Here's how the part is built. I have some questions about the finished solid (model axes, mm). A direction names the side the tool comes from. Coordinates: 2 decimals unless noted, no trailing zeros. Write each loop counter-clockwise with the first axis right and the second up, starting at its lowest first coordinate (ties: lowest second). Pieces come first, ordered by that corner, then holes. Notation, with made-up numbers: (-6, 16.25) -> (5, 16.25) arc R17 cw to (5, 28.25) -> close; hole circle Ø8 at (44.5, 6). An arc over 180 degrees is marked (long way). Put each result on its own line as item: value. Start each with the question number.
Item 1: I want a section at D-D, the plane x = 9. List the corners of the cut face in (y, z) for me, then the cut area to 3 significant figures.
Item 2: If we mould it in two halves opening along Y, with no side actions, what happens to faces 5 (the face through (0, 108, -20)), 6 (the face through (0, 99, -23)), 7 (the face through (0, 15, -8))? For each: released by +Y, released by -Y, zero draft, split by the parting line, or undercut.
Item 3: On a 3-axis mill with a long thin cutter (end or side, diameter ignored), from which of +Z, -Z, +X, -X, +Y, -Y can I reach the whole of each face in a straight line? I mean faces 1 (the face through (20, 35, -16)), 2 (the face through (-17.5, 56, -8)), 3 (the face through (25.65, 102.17, -5.07)), 4 (the face through (-23.34, 53.24, -4.31)). Say none if no direction works.
Item 4: I want a section at B-B, the plane x = 19.5. List the corners of the cut face in (y, z) for me.
Item 5: I want a section at A-A, the plane y = 63.5. List the corners of the cut face in (x, z) for me, then the cut area to 3 significant figures.
Item 6: I need wall thicknesses on line 1 (X direction, y = 100, z = -5); line 2 (X direction, y = 52, z = -4.5); line 3 (X direction, y = 74, z = -10). Which ranges of each line are inside material? Lowest first, please. Write a range as [from, to].
Item 7: I want a section at C-C, the plane y = 10. List the corners of the cut face in (x, z) for me.
Item 8: For pin 1 (4 mm diameter, centred on x = 3.5, z = -36, fed in from -Y); pin 2 (6.5 mm diameter, centred on x = -19.5, y = 10, fed in from -Z), each with a flat end and sliding along its axis, tell me the tip position at first contact or that it passes through.
from build123d import *

# Parameters (mm, degrees)
EXTRUDE_2_DEPTH        = 29.5
HOLE_WIZARD_M4_2_D     = 3.3
HOLE_WIZARD_M4_2_DEPTH = 11.5
HOLE_WIZARD_M4_2_TIP   = 0.991420021
CUT_EXTRUDE_1_DEPTH    = 119.887551914
HOLE_WIZARD_M5_1_D     = 4.2
HOLE_WIZARD_M3_1_D     = 2.5
HOLE_WIZARD_M3_1_DEPTH = 8.5
HOLE_WIZARD_M3_1_TIP   = 0.751075774
HOLE_WIZARD_M4_3_D     = 3.3
HOLE_WIZARD_M4_3_DEPTH = 11.5
HOLE_WIZARD_M4_3_TIP   = 0.991420021


with BuildPart() as part:
    # 草图5 → 凸台-拉伸2 (new, symmetric)
    with BuildSketch(Plane(origin=(0, 0, 0), x_dir=(0, 0, -1), z_dir=(1, 0, 0))):
        Polygon((26, 102), (40, 102), (40, 108), (0, 108), (0, 0), (16, 0), (16, 92), align=None)
    extrude(amount=EXTRUDE_2_DEPTH, both=True)

    # M4 螺纹孔2
    with Locations(Plane(origin=(0, 108, 0), x_dir=(1, 0, 0), z_dir=(0, 1, 0))):
        with Locations((24, 5), (-24, 5)):
            Hole(HOLE_WIZARD_M4_2_D / 2, depth=HOLE_WIZARD_M4_2_DEPTH)
            with Locations((0, 0, -(HOLE_WIZARD_M4_2_DEPTH + HOLE_WIZARD_M4_2_TIP / 2))):  # 118° drill point
                Cone(0, HOLE_WIZARD_M4_2_D / 2, HOLE_WIZARD_M4_2_TIP, mode=Mode.SUBTRACT)

    # 草图8 → 切除-拉伸1 (cut, through all)
    with BuildSketch(Plane.XY):
        with BuildLine():
            Line((17.5, 80.5), (17.5, 32.5))
            ThreePointArc((17.5, 32.5), (0, 15), (-17.5, 32.5))
            Line((-17.5, 32.5), (-17.5, 80.5))
            ThreePointArc((-17.5, 80.5), (0, 98), (17.5, 80.5))
        make_face()
    extrude(amount=-CUT_EXTRUDE_1_DEPTH, mode=Mode.SUBTRACT)

    # M5 螺纹孔1 (through all)
    with Locations(Plane.XY):
        with Locations((-19.5, 10), (19.5, 10)):
            Hole(HOLE_WIZARD_M5_1_D / 2)

    # M3 螺纹孔1
    with Locations(Plane.XY):
        with Locations((23.5, 42), (-23.5, 52), (-23.5, 42), (23.5, 52)):
            Hole(HOLE_WIZARD_M3_1_D / 2, depth=HOLE_WIZARD_M3_1_DEPTH)
            with Locations((0, 0, -(HOLE_WIZARD_M3_1_DEPTH + HOLE_WIZARD_M3_1_TIP / 2))):  # 118° drill point
                Cone(0, HOLE_WIZARD_M3_1_D / 2, HOLE_WIZARD_M3_1_TIP, mode=Mode.SUBTRACT)

    # M4 螺纹孔3
    with Locations(Plane(origin=(0, 0, 0), x_dir=(-1, 0, 0), z_dir=(0, -1, 0))):
        with Locations((0, 8)):
            Hole(HOLE_WIZARD_M4_3_D / 2, depth=HOLE_WIZARD_M4_3_DEPTH)
            with Locations((0, 0, -(HOLE_WIZARD_M4_3_DEPTH + HOLE_WIZARD_M4_3_TIP / 2))):  # 118° drill point
                Cone(0, HOLE_WIZARD_M4_3_D / 2, HOLE_WIZARD_M4_3_TIP, mode=Mode.SUBTRACT)


solid = part.part
Calculated:
1. outline: (0, -16) -> (17.49, -16) -> (17.49, 0) -> (0, 0) -> close; (95.51, -19.51) -> (102, -26) -> (102, -40) -> (108, -40) -> (108, 0) -> (95.51, 0) -> close
1. area: 668 mm2
2. face 5: released by +Y
2. face 6: released by -Y
2. face 7: undercut
3. face 1: -Z, +X, -X, -Y
3. face 2: +Z, -Z
3. face 3: +Y
3. face 4: +Z
4. outline: (0, -16) -> (7.9, -16) -> (7.9, 0) -> (0, 0) -> close; (12.1, -16) -> (92, -16) -> (102, -26) -> (102, -40) -> (108, -40) -> (108, 0) -> (12.1, 0) -> close
5. outline: (-29.5, -16) -> (-17.5, -16) -> (-17.5, 0) -> (-29.5, 0) -> close; (17.5, -16) -> (29.5, -16) -> (29.5, 0) -> (17.5, 0) -> close
5. area: 384 mm2
6. line 1: x = [-29.5, -25.65], [-22.35, 22.35], [25.65, 29.5]
6. line 2: x = [-29.5, -24.75], [-22.25, -17.5], [17.5, 22.25], [24.75, 29.5]
6. line 3: x = [-29.5, -17.5], [17.5, 29.5]
7. outline: (-29.5, -16) -> (-21.6, -16) -> (-21.6, 0) -> (-29.5, 0) -> close; (-17.4, -16) -> (17.4, -16) -> (17.4, 0) -> (-17.4, 0) -> close; (21.6, -16) -> (29.5, -16) -> (29.5, 0) -> (21.6, 0) -> close; hole circle Ø3.3 at (0, -8)
8. pin 1: stops at y = 102
8. pin 2: stops at z = -16
